Verification items for the finished model (mm, model axes). A direction names the side the tool comes from. Round coordinates to 2 decimals unless told otherwise and drop trailing zeros. Order: outer loops, then holes, each group sorted by start corner. A loop starts at its lowest first (then second) coordinate and runs counter-clockwise, first axis right, second up. Notation, with made-up numbers: M 85,-36 L 125,-36 A15 ccw 125,-17 Z; hole C 4,44.25 d2. An arc over 180 degrees is marked long. Answer as a JSON object with one key per item and string values. Group by question number.
```python
from build123d import *

# Parameters (mm, degrees)
CHAMFER_1_SIZE = 1


with BuildPart() as part:
    # 草图1 → 旋转1 (revolve)
    with BuildSketch(Plane(origin=(0, 0, 0), x_dir=(0, 0, -1), z_dir=(1, 0, 0)), mode=Mode.PRIVATE) as revolve_1_sk:
        Polygon((79.5, 2.5), (2, 2.5), (2, 3.5), (0, 3.5), (0, 0), (82.3, 0), (82.3, 2.5), (80.3, 2.5), (80.3, 1.75), (79.5, 1.75), align=None)
    revolve(revolve_1_sk.sketch.rotate(Axis((0, 0, 0), (0, 0, -1)), 90), axis=Axis((0, 0, 0), (0, 0, -1)))

    # 倒角1
    chamfer_1_edges = [part.edges().sort_by_distance(p)[0] for p in [
        (-2.5, 0, -82.3),
    ]]
    chamfer(chamfer_1_edges, length=CHAMFER_1_SIZE)


solid = part.part
```
Q1. Cross-section at A-A, the plane x = 0. Record the cut outline in (y, z).
Q2. Gauge pin test, flat ends, axial feed: pin 1 Ø2 at (x, y) = (1.5, 0.5) entering from -Z; pin 2 Ø4 at (x, z) = (0, -49) entering from +Y; pin 3 Ø1.5 at (x, y) = (-2.5, -1) entering from -Z; pin 4 Ø1 at (x, z) = (1, -19.5) entering from +Y. Record the tip position at first contact, or that the pin passes through.
Q3. Tool access check on faces 1 (the face through (1, -2, -80.3)), 2 (the face through (-2.5, -0.1, -80.8)), 3 (the face through (0, 0, 0)). Record the directions out of +Z, -Z, +X, -X, +Y, -Y that give a thin tool (end or side, any length) a straight path to the whole face; none if there is none.
Q4. Thickness scan on line 1 (Z direction, x = 2.5, y = -1.75); line 2 (X direction, y = 2, z = -70.5); line 3 (Z direction, x = 2.25, y = -0.5). Record the ranges inside material, lowest first. Write a range as from..to.
Q5. Cross-section at C-C, the plane z = -67. Record the cut outline in (x, y), then the cut area to 3 significant figures.
Q6. Release check for a two-part mould opening along Z. For faces 4 (the face through (-1, -2, -79.5)), 5 (the face through (0.81, 1.55, -79.89)), 6 (the face through (1.615, 3.105, -0.986)), 7 (the face through (-2, 2, -2)) record: released by +Z, released by -Z, zero draft, split by the parting line, or undercut.
Conclusion:
{
 "1": {"outline": "M -3.5,-2 L -2.5,-2 L -2.5,-79.5 L -1.75,-79.5 L -1.75,-80.3 L -2.5,-80.3 L -2.5,-81.3 L -1.5,-82.3 L 1.5,-82.3 L 2.5,-81.3 L 2.5,-80.3 L 1.75,-80.3 L 1.75,-79.5 L 2.5,-79.5 L 2.5,-2 L 3.5,-2 L 3.5,0 L -3.5,0 Z"},
 "2": {"pin 1": "z = -82.3", "pin 2": "y = 2.5", "pin 3": "z = -81.86", "pin 4": "y = 2.45"},
 "3": {"face 1": "none", "face 2": "-Z", "face 3": "+Z, +X, -X, +Y, -Y"},
 "4": {"line 1": "-2..0", "line 2": "-1.5..1.5", "line 3": "-81.5..-80.3, -79.5..0"},
 "5": {"outline": "C 0,0 d5", "area": "19.6 mm2"},
 "6": {"face 4": "undercut", "face 5": "undercut", "face 6": "zero draft", "face 7": "released by -Z"}
}
